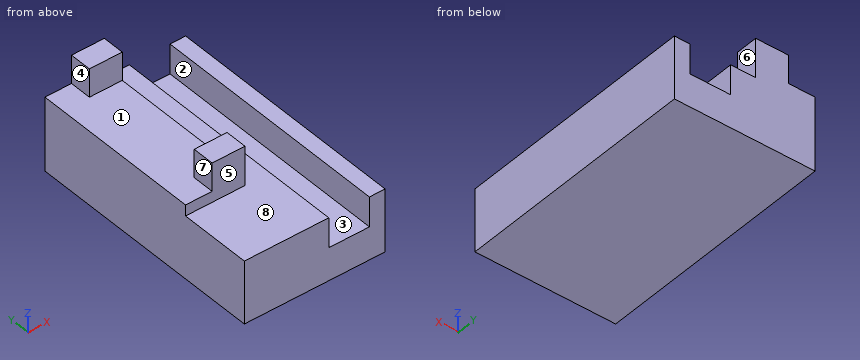
```python
from build123d import *

# Parameters (mm, degrees)
SKETCH4_W           = 45
SKETCH4_H           = 78
BOSS_EXTRUDE1_DEPTH = 20
SKETCH6_W           = 13
SKETCH6_H           = 9.5
CUT_EXTRUDE1_DEPTH  = 86.511276786
SKETCH7_W           = 10.5
SKETCH7_H           = 55
BOSS_EXTRUDE2_DEPTH = 3.5
SKETCH8_W           = 10.5
SKETCH8_H           = 7
BOSS_EXTRUDE3_DEPTH = 9
SKETCH9_W           = 8.5
SKETCH9_H           = 55
BOSS_EXTRUDE4_DEPTH = 3.5


with BuildPart() as part:
    # Sketch4 → Boss-Extrude1 (new body)
    with BuildSketch(Plane.XY):
        with Locations((-6.278089888, 16.575842697)):
            Rectangle(SKETCH4_W, SKETCH4_H)
    extrude(amount=BOSS_EXTRUDE1_DEPTH)

    # Sketch6 → Cut-Extrude1 (cut, through all)
    with BuildSketch(Plane.XZ.offset(22.424157303)):
        with Locations((4.721910112, 15.25)):
            Rectangle(SKETCH6_W, SKETCH6_H)
    extrude(amount=-CUT_EXTRUDE1_DEPTH, mode=Mode.SUBTRACT)

    # Sketch7 → Boss-Extrude2 (add)
    with BuildSketch(Plane.XY.offset(20)):
        with Locations((-15.028089888, 28.075842697)):
            Rectangle(SKETCH7_W, SKETCH7_H)
    extrude(amount=BOSS_EXTRUDE2_DEPTH)

    # Sketch8 → Boss-Extrude3 (add)
    with BuildSketch(Plane.XY.offset(23.5)):
        with Locations((-15.028089888, 4.075842697)):
            Rectangle(SKETCH8_W, SKETCH8_H)
        with Locations((-15.028089888, 52.075842697)):
            Rectangle(SKETCH8_W, SKETCH8_H)
    extrude(amount=BOSS_EXTRUDE3_DEPTH)

    # Sketch9 → Boss-Extrude4 (add)
    with BuildSketch(Plane.XY.offset(20)):
        with Locations((-24.528089888, 28.075842697)):
            Rectangle(SKETCH9_W, SKETCH9_H)
    extrude(amount=BOSS_EXTRUDE4_DEPTH)


solid = part.part
```
The model under review builds one solid part; all positions refer to its coordinate system, in mm. Face numbers are marked on the shaded views. A direction names the side the tool comes from. Coordinates: 2 decimals unless noted, no trailing zeros. Write each loop counter-clockwise with the first axis right and the second up, starting at its lowest first coordinate (ties: lowest second). Pieces come first, ordered by that corner, then holes. Notation, with made-up numbers: (4, 2) - (41, 2) arc R20 ccw to (41, 17) - close; hole circle Ø4 at (54.25, -6.75). An arc over 180 degrees is marked (long way). Answer in a Markdown table with one row per item. Add a question column.
Q1. Draft analysis for pull direction X (two halves, no side actions). For the marked faces 1, 2, 3 and 4, state which applies: +X half, -X half, draft (parallel to the pull), parting line (faces both ways), or undercut.
Q2. Consider section D-D on z = 12.5. Give the boundary of the cut face in (x, y).
Q3. For the marked faces 5, 6, 7 and 8, list the 3-axis set-ups (+Z, -Z, +X, -X, +Y, -Y) from which the entire face can be reached by the end or side of a thin tool; tool diameter is ignored.
Q4. Consider section B-B on x = -19. Give the boundary of the cut face in (y, z).
Q5. Clearance check with flat-ended pins moving along their axes: pin 1 (4 mm diameter, centred on x = -21, z = 28, fed in from -Y); pin 2 (14.5 mm diameter, centred on x = 3.5, y = 12, fed in from +Z); pin 3 (15 mm diameter, centred on x = -17.5, y = 36.5, fed in from +Z). State where each tip first meets the part, or that it passes through.
Q6. Consider section A-A on z = 29.5. Give the boundary of the cut face in (x, y), then the cut area to 3 significant figures.
Q7. To check wall thickness, follow line 1 along X through (y, z) = (15.5, 17); line 2 along Y through (x, z) = (-16, 25); line 3 along Z through (x, y) = (9.5, -12). State the ranges of each line that lie inside material, in increasing order. Write a range as from..to.
Q8. Consider section C-C on y = 10. Give the boundary of the cut face in (x, z).
Answers below:
| question | item | result |
|---|---|---|
| 1 | face 1 | draft |
| 1 | face 2 | undercut |
| 1 | face 3 | undercut |
| 1 | face 4 | -X half |
| 2 | outline | (-28.78, -22.42) - (-1.78, -22.42) - (-1.78, 55.58) - (-28.78, 55.58) - close; (11.22, -22.42) - (16.22, -22.42) - (16.22, 55.58) - (11.22, 55.58) - close |
| 3 | face 5 | +Z, +X, -X, -Y |
| 3 | face 6 | +Z, +X, +Y, -Y |
| 3 | face 7 | +Z, -X, +Y, -Y |
| 3 | face 8 | +Z, +X, -Y |
| 4 | outline | (-22.42, 0) - (55.58, 0) - (55.58, 32.5) - (48.58, 32.5) - (48.58, 23.5) - (7.58, 23.5) - (7.58, 32.5) - (0.58, 32.5) - (0.58, 20) - (-22.42, 20) - close |
| 5 | pin 1 | y = 0.58 |
| 5 | pin 2 | z = 20 |
| 5 | pin 3 | z = 23.5 |
| 6 | outline | (-20.28, 0.58) - (-9.78, 0.58) - (-9.78, 7.58) - (-20.28, 7.58) - close; (-20.28, 48.58) - (-9.78, 48.58) - (-9.78, 55.58) - (-20.28, 55.58) - close |
| 6 | area | 147 mm² |
| 7 | line 1 | -28.78..-1.78, 11.22..16.22 |
| 7 | line 2 | 0.58..7.58, 48.58..55.58 |
| 7 | line 3 | 0..10.5 |
| 8 | outline | (-28.78, 0) - (16.22, 0) - (16.22, 20) - (11.22, 20) - (11.22, 10.5) - (-1.78, 10.5) - (-1.78, 20) - (-9.78, 20) - (-9.78, 23.5) - (-28.78, 23.5) - close |
